Can you work these out from the model? Positions are in its coordinate system, mm. Face numbers are marked on the shaded views. A direction names the side the tool comes from. Round coordinates to 2 decimals unless told otherwise and drop trailing zeros. Loops run counter-clockwise (first coordinate to the right, second up) from the corner with the lowest first, then second, coordinate; pieces in that order, holes last. Notation, with made-up numbers: (81.5, 81.5) -> (128.5, 81.5) arc R23 ccw to (128.5, 99.5) -> close; hole circle Ø6 at (34.25, 64). An arc over 180 degrees is marked (long way). Write each question's results on one line, items separated by ' | '.
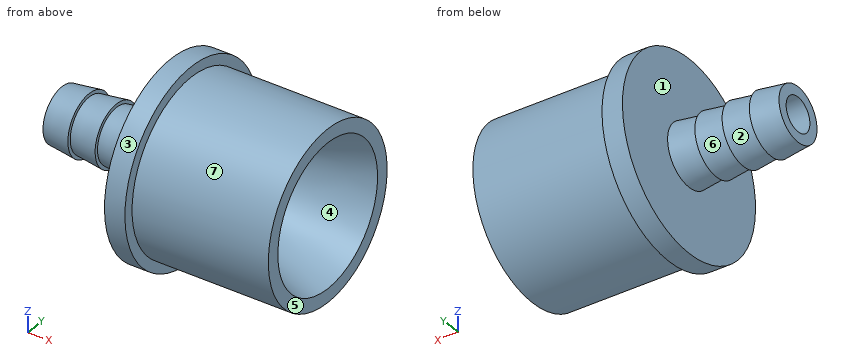
from build123d import *


with BuildPart() as part:
    # Esboço1 → Revolução1 (revolve)
    with BuildSketch(Plane.XY, mode=Mode.PRIVATE) as revolu_o1_sk:
        Polygon((-27.323427807, 14), (-27.323427807, 12.5), (-7.323427807, 12.5), (-7.323427807, 10.5), (-29.115185999, 2.5), (-46.323427807, 2.5), (-46.323427807, 4), (-42.323427807, 4.5), (-42.323427807, 4), (-38.323427807, 4.5), (-38.323427807, 4), (-34.323427807, 4.5), (-34.323427807, 4), (-30.323427807, 4.5), (-30.323427807, 14), align=None)
    revolve(revolu_o1_sk.sketch.rotate(Axis((48.321734693, 0, 0), (-1, 0, 0)), 90), axis=Axis((48.321734693, 0, 0), (-1, 0, 0)))


solid = part.part
1. On a 3-axis mill with a long thin cutter (end or side, diameter ignored), from which of +Z, -Z, +X, -X, +Y, -Y can I reach the whole of each face in a straight line? I mean the marked faces 5, 6 and 7. Say none if no direction works.
Final values:
face 5: +Z, -Z, +X, +Y, -Y | face 6: none | face 7: +X
2. Please list where these lines run through material, in increasing order: line 1 (Y direction, x = -34.25, z = 0); line 2 (X direction, y = 10.25, z = -7); line 3 (Z direction, x = -14, y = 5.25). Write a range as from..to.
Final values:
line 1: -4.01..-2.5, 2.5..4.01 | line 2: -30.32..-7.32 | line 3: -11.34..-6.1, 6.1..11.34
3. If we section it at C-C (x = -32.5): List the corners of the cut face in (y, z) for me.
Final values:
outline: circle Ø8.46 at (0, 0); hole circle Ø5 at (0, 0)
4. Will these pins go through, and if not, where does the flat tip stop? pin 1 (6 mm diameter, centred on x = -15, y = 5.5, fed in from -Z); pin 2 (5 mm diameter, centred on x = -33.5, y = -4, fed in from -Z); pin 3 (5 mm diameter, centred on x = -16, z = -8.5, fed in from +Y).
Final values:
pin 1: z = -12.25 | pin 2: z = -4.19 | pin 3: y = 10.97
5. We'd pull the mould along X, two halves only. Please class the marked faces 1, 2, 3 and 4: pulls with the +X half, pulls with the -X half, needs draft (parallel to the pull), parting line crosses it, or undercut.
Final values:
face 1: pulls with the -X half | face 2: undercut | face 3: needs draft | face 4: pulls with the +X half
